```python
from build123d import *

# Parameters (mm, degrees)
F0_R          = 100
F0_R_2        = 30
F1_DEPTH      = 5
F0_R_3        = 27.5
F2_DEPTH      = 5
F2_DEPTH_BACK = 66
F3_START      = -61
F3_DEPTH      = 5


with BuildPart() as f1:
    # F0 (on Top) → F1 (new body)
    with BuildSketch(Plane.XY):
        Circle(F0_R)
        Circle(F0_R_2, mode=Mode.SUBTRACT)
    extrude(amount=F1_DEPTH)

    # F0 (on Top) → F2 (join, two sides)
    with BuildSketch(Plane.XY) as f2_sk:
        Circle(F0_R_2)
        Circle(F0_R_3, mode=Mode.SUBTRACT)
    extrude(amount=F2_DEPTH)
    extrude(f2_sk.sketch, amount=-F2_DEPTH_BACK)

    # F0 (on Top) → F3 (join)
    with BuildSketch(Plane.XY.offset(F3_START)):
        Circle(F0_R)
        Circle(F0_R_2, mode=Mode.SUBTRACT)
    extrude(amount=-F3_DEPTH)


solid = f1.part
```
The listing builds one solid part. Answer for the finished solid, in the listing's coordinates (mm). A direction names the side the tool comes from. Give positions to 0.01 mm unless a question says otherwise; leave off trailing zeros. Loops run counter-clockwise (first coordinate to the right, second up) from the corner with the lowest first, then second, coordinate; pieces in that order, holes last. Notation, with made-up numbers: M 15,-7.75 L 67,-7.75 A31 cw 67,18.25 Z; hole C 36.5,-27.75 d8. An arc over 180 degrees is marked long. One line per item, written item: value.
Q1. Determine the mould class of faces 3 (the face through (21, -21, 5)), 4 (the face through (95.38, 30.04, 2.46)), 5 (the face through (-24, -21, -61)) for opening direction Z: +Z half, -Z half, draft (parallel to the pull), parting line (faces both ways), or undercut.
Working result:
face 3: +Z half
face 4: draft
face 5: undercut
Q2. A cutting plane is placed at B-B on x = 60. Determine the outline of the cut face in (y, z).
Working result:
outline: M -80,-66 L 80,-66 L 80,-61 L -80,-61 Z; M -80,0 L 80,0 L 80,5 L -80,5 Z
Q3. A cutting plane is placed at D-D on z = -34. Determine the outline of the cut face in (x, y).
Working result:
outline: C 0,0 d60; hole C 0,0 d55
Q4. Find the intervals of material crossed by line 1 (Y direction, x = 0, z = -37); line 2 (Z direction, x = 67, y = -67); line 3 (Y direction, x = 0, z = 2), in increasing order. Write a range as from..to.
Working result:
line 1: y = -30..-27.5, 27.5..30
line 2: z = -66..-61, 0..5
line 3: y = -100..-27.5, 27.5..100
Q5. For faces 1 (the face through (21, 24, 0)), 2 (the face through (21, -21, -66)), determine the directions among +Z, -Z, +X, -X, +Y, -Y from which every point of the face is accessible in a straight line to the end or side of a thin tool.
Working result:
face 1: none
face 2: -Z, +X, -X, +Y, -Y
Q6. A cutting plane is placed at A-A on y = 0. Determine the outline of the cut face in (x, z).
Working result:
outline: M -100,-66 L -27.5,-66 L -27.5,5 L -100,5 L -100,0 L -30,0 L -30,-61 L -100,-61 Z; M 27.5,-66 L 100,-66 L 100,-61 L 30,-61 L 30,0 L 100,0 L 100,5 L 27.5,5 Z
Q7. A flat-ended cylindrical pin translates along its axis: P1, Ø8, axis at x = 11.5, z = -54, coming from the +Y side. Find the tip coordinate at first contact, or state that the pin passes through.
Working result:
P1: stops at y = 29.05
